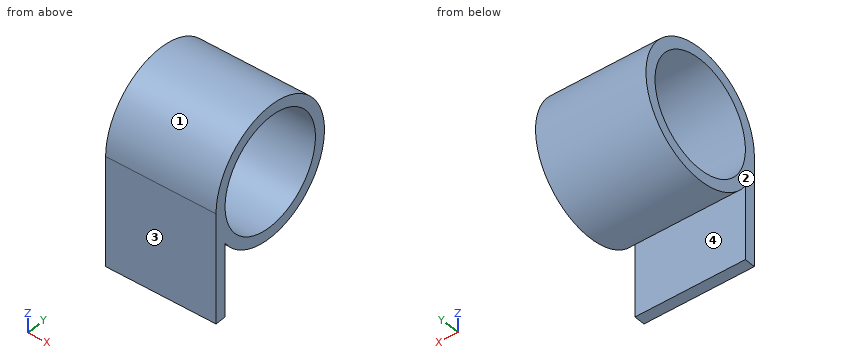
```python
from build123d import *

# Parameters (mm, degrees)
SKETCH1_R           = 5
BOSS_EXTRUDE1_DEPTH = 10


with BuildPart() as part:
    # Sketch1 → Boss-Extrude1 (new body)
    with BuildSketch(Plane(origin=(0, 0, 0), x_dir=(0, 0, -1), z_dir=(1, 0, 0))):
        with BuildLine():
            Line((10, -5), (3.31662479, -5))
            ThreePointArc((3.31662479, -5), (-1.732050808, 5.744562647), (0, -6))
            Line((0, -6), (10, -6))
            Line((10, -6), (10, -5))
        make_face()
        Circle(SKETCH1_R, mode=Mode.SUBTRACT)
    extrude(amount=BOSS_EXTRUDE1_DEPTH)


solid = part.part
```
Source: CAD feature listing. Evaluate the final solid. Frame: model axes, mm. Face numbers are marked on the shaded views. Round coordinates to 2 decimals unless told otherwise and drop trailing zeros. Loops run counter-clockwise (first coordinate to the right, second up) from the corner with the lowest first, then second, coordinate; pieces in that order, holes last. Notation, with made-up numbers: M 34.5,86 L 52.5,86 A17 cw 52.5,97 Z; hole C -20.5,9.25 d11. An arc over 180 degrees is marked long. Use a Markdown table: item, result. Add a question column.
1. Cut plane C-C, the plane x = 0.5. Output: boundary loops of the cut face in (y, z), and give its area (3 significant figures).
2. Cut plane B-B, the plane z = -1.75. Output: boundary loops of the cut face in (x, y).
3. Cut plane A-A, the plane y = 0. Output: boundary loops of the cut face in (x, z), and give its area (3 significant figures).
4. Cut plane D-D, the plane z = -4. Output: boundary loops of the cut face in (x, y).
5. Pull-direction query (Y, two-part tool) for the marked faces 1, 2, 3 and 4; classes: +Y half, -Y half, draft (parallel to the pull), parting line (faces both ways), or undercut.
6. Contact query for flat-ended pins moving along their axis: pin 1 (1 mm diameter, centred on y = 1, z = 2.5, fed in from +X); pin 2 (6 mm diameter, centred on x = 1.5, z = 4.5, fed in from -Y); pin 3 (5 mm diameter, centred on x = 3, y = 0, fed in from -Z). Output: stop coordinate, or through.
7. Ray query, line 1 along Z through (x, y) = (6, -3.25); line 2 along Z through (x, y) = (7.5, -1); line 3 along Y through (x, z) = (5.75, 3.75). Return the intervals inside material, ascending. Write a range as [from, to].
Solution:
| question | item | result |
|---|---|---|
| 1 | outline | M -6,-10 L -5,-10 L -5,-3.32 A6 ccw long -6,0 Z; hole C 0,0 d10 |
| 1 | area | 42.3 mm2 |
| 2 | outline | M 0,-6 L 10,-6 L 10,-4.68 L 0,-4.68 Z; M 0,4.68 L 10,4.68 L 10,5.74 L 0,5.74 Z |
| 3 | outline | M 0,-6 L 10,-6 L 10,-5 L 0,-5 Z; M 0,5 L 10,5 L 10,6 L 0,6 Z |
| 3 | area | 20.0 mm2 |
| 4 | outline | M 0,-6 L 10,-6 L 10,-5 L 0,-5 Z; M 0,-4.47 L 10,-4.47 L 10,-3 L 0,-3 Z; M 0,3 L 10,3 L 10,4.47 L 0,4.47 Z |
| 5 | face 1 | undercut |
| 5 | face 2 | draft |
| 5 | face 3 | -Y half |
| 5 | face 4 | undercut |
| 6 | pin 1 | passes through |
| 6 | pin 2 | stops at y = -5.81 |
| 6 | pin 3 | stops at z = -6 |
| 7 | line 1 | z = [-5.04, -3.8], [3.8, 5.04] |
| 7 | line 2 | z = [-5.92, -4.9], [4.9, 5.92] |
| 7 | line 3 | y = [-4.68, -3.31], [3.31, 4.68] |
